CAD build for the part. Positions are in the model's coordinates, mm. A direction names the side the tool comes from. Round coordinates to 2 decimals unless told otherwise and drop trailing zeros. Write each loop counter-clockwise with the first axis right and the second up, starting at its lowest first coordinate (ties: lowest second). Pieces come first, ordered by that corner, then holes. Notation, with made-up numbers: (12.25, 60) -> (33.25, 60) arc R10 ccw to (33.25, 74) -> close; hole circle Ø10 at (56, 49.25). An arc over 180 degrees is marked (long way). Put each result on its own line as item: value. Start each with the question number.
1. Drill centre lines: line 1 (X direction, y = 12.5, z = 46.25); line 2 (X direction, y = -6.5, z = 46.25); line 3 (Y direction, x = 8, z = 40.25). Where is each one in solid material? Low to high. Write a range as from..to.
2. Saw through at C-C on z = 35. List the corners of the cut face in (x, y).
3. Saw through at B-B on x = 0. List the corners of the cut face in (y, z), and give its area (3 significant figures).
4. 3-axis set-ups, long thin cutter, end or side, ignore diameter. For faces 4 (the flat face through (13, 7, 47)), 5 (the flat face through (-9, 0, 41.5)), 6 (the flat face through (-13, 7, 47)), 7 (the flat face through (-11, -7, 39)), 8 (the cylindrical face through (6.384, 7.721, 46.43)): which of +Z, -Z, +X, -X, +Y, -Y reach the whole face in a straight line?
5. Flat gauge pins, fed straight in: P1, Ø15, axis at x = 0, y = -6.5, coming from the -Z side; P2, Ø3, axis at y = 2.5, z = 45, coming from the +X side; P3, Ø1.5, axis at x = -4.5, y = -5, coming from the -Z side; P4, Ø1, axis at x = -5.5, z = 37.5, coming from the +Y side. Where does each tip first touch, or does it go through?
6. Pull direction Z, two halves, no side cores. Call faces 1 (the flat face through (-10, 0, 51.5)), 2 (the flat face through (0, -14, 33)), 3 (the flat face through (12, 0, 46)): pulls with the +Z half, pulls with the -Z half, needs draft (parallel to the pull), parting line crosses it, or undercut.
7. Saw through at D-D on y = -23. List the corners of the cut face in (x, z), and give its area (3 significant figures).
8. Saw through at A-A on y = 0. List the corners of the cut face in (x, z).
from build123d import *

# Parameters (mm, degrees)
BOX005_W                  = 12
BOX005_H                  = 60
BOX005_DEPTH              = 30
BOX006_W                  = 12
BOX006_H                  = 60
BOX006_DEPTH              = 30
BOX004_W                  = 50
BOX004_H                  = 30
BOX004_DEPTH              = 19
BOX004_PLACEMENT_ANGLE    = 15
CYLINDER012_R             = 5.1
CYLINDER012_DEPTH         = 50
CYLINDER007_R             = 7.5
CYLINDER007_DEPTH         = 70
CYLINDER009_R             = 6.5
CYLINDER009_DEPTH         = 70
CYLINDER010_R             = 7.5
CYLINDER010_DEPTH         = 70
CYLINDER011_R             = 6.5
CYLINDER011_DEPTH         = 70
FUSION007_PLACEMENT_ANGLE = 180
CYLINDER008_R             = 5.1
CYLINDER008_DEPTH         = 70
BOX003_W                  = 57
BOX003_H                  = 59
BOX003_DEPTH              = 20
CYLINDER004_R             = 6.35
CYLINDER004_DEPTH         = 50
BOX_W                     = 40
BOX_H                     = 20
BOX_DEPTH                 = 30
BOX_PLACEMENT_ANGLE       = 15
CYLINDER001_R             = 5
CYLINDER001_DEPTH         = 50
CYLINDER006_R             = 6.35
CYLINDER006_DEPTH         = 50
BOX001_W                  = 40
BOX001_H                  = 20
BOX001_DEPTH              = 30
BOX001_PLACEMENT_ANGLE    = 15
CYLINDER005_R             = 5
CYLINDER005_DEPTH         = 50
FUSION003_PLACEMENT_ANGLE = 180
BOX002_W                  = 24
BOX002_H                  = 39
BOX002_DEPTH              = 10


with BuildPart() as cube005:
    # Box005 → Box005 (new body)
    with BuildSketch(Plane(origin=(14, -29, 23), x_dir=(1, 0, 0), z_dir=(0, 0, 1))):
        with Locations((6, 30)):
            Rectangle(BOX005_W, BOX005_H)
    extrude(amount=BOX005_DEPTH)


with BuildPart() as fusion009:
    # Box006 → Box006 (new body)
    with BuildSketch(Plane(origin=(-26, -29, 23), x_dir=(1, 0, 0), z_dir=(0, 0, 1))):
        with Locations((6, 30)):
            Rectangle(BOX006_W, BOX006_H)
    extrude(amount=BOX006_DEPTH)

    # Fusion009: union Cube005
    add(cube005.part)


with BuildPart() as cube004:
    # Box004 → Box004 (new body)
    with BuildSketch(Plane.XY):
        with Locations((25, 15)):
            Rectangle(BOX004_W, BOX004_H)
    extrude(amount=BOX004_DEPTH)


with BuildPart() as cube004_1:
    # Box004 placement: moved
    add(cube004.part.moved(Location((-24, 7.965926, 22.258819))).rotate(Axis((-24, 7.965926, 22.258819), (1, 0, 0)), BOX004_PLACEMENT_ANGLE))


with BuildPart() as obj1:
    # Cylinder012 → Cylinder012 (new body)
    with BuildSketch(Plane(origin=(0, -12.5, -17), x_dir=(1, 0, 0), z_dir=(0, 0, 1))):
        Circle(CYLINDER012_R)
    extrude(amount=CYLINDER012_DEPTH)


with BuildPart() as obj2:
    # Cylinder007 → Cylinder007 (new body)
    with BuildSketch(Plane.XY):
        Circle(CYLINDER007_R)
    extrude(amount=CYLINDER007_DEPTH)


with BuildPart() as fusion006:
    # Cylinder009 → Cylinder009 (new body)
    with BuildSketch(Plane(origin=(0, 6.5, 0), x_dir=(1, 0, 0), z_dir=(0, 0, 1))):
        Circle(CYLINDER009_R)
    extrude(amount=CYLINDER009_DEPTH)

    # Fusion006: union obj2
    add(obj2.part)


with BuildPart() as obj3:
    # Cylinder010 → Cylinder010 (new body)
    with BuildSketch(Plane.XY):
        Circle(CYLINDER010_R)
    extrude(amount=CYLINDER010_DEPTH)


with BuildPart() as fusion008:
    # Cylinder011 → Cylinder011 (new body)
    with BuildSketch(Plane(origin=(0, 6.5, 0), x_dir=(1, 0, 0), z_dir=(0, 0, 1))):
        Circle(CYLINDER011_R)
    extrude(amount=CYLINDER011_DEPTH)

    # Fusion007: union obj3
    add(obj3.part)


with BuildPart() as fusion008_1:
    # Fusion007 placement: moved
    add(fusion008.part.rotate(Axis((0, 0, 0), (0, 0, 1)), FUSION007_PLACEMENT_ANGLE))

    # Fusion008: union Fusion006
    add(fusion006.part)


with BuildPart() as cylinder008:
    # Cylinder008 → Cylinder008 (new body)
    with BuildSketch(Plane(origin=(0, 12.5, 0), x_dir=(1, 0, 0), z_dir=(0, 0, 1))):
        Circle(CYLINDER008_R)
    extrude(amount=CYLINDER008_DEPTH)


with BuildPart() as cube003:
    # Box003 → Box003 (new body)
    with BuildSketch(Plane(origin=(-29.5, -29, 51.5), x_dir=(1, 0, 0), z_dir=(0, 0, 1))):
        with Locations((28.5, 29.5)):
            Rectangle(BOX003_W, BOX003_H)
    extrude(amount=BOX003_DEPTH)


with BuildPart() as obj4:
    # Cylinder004 → Cylinder004 (new body)
    with BuildSketch(Plane.XY):
        Circle(CYLINDER004_R)
    extrude(amount=CYLINDER004_DEPTH)


with BuildPart() as cube:
    # Box → Box (new body)
    with BuildSketch(Plane.XY):
        with Locations((20, 10)):
            Rectangle(BOX_W, BOX_H)
    extrude(amount=BOX_DEPTH)


with BuildPart() as cube_1:
    # Box placement: moved
    add(cube.part.moved(Location((-19.558238, 7, 39.759763))).rotate(Axis((-19.558238, 7, 39.759763), (0, 1, 0)), BOX_PLACEMENT_ANGLE))


with BuildPart() as fusion001:
    # Cylinder001 → Cylinder001 (new body)
    with BuildSketch(Plane(origin=(0, 12.5, 0), x_dir=(1, 0, 0), z_dir=(0, 0, 1))):
        Circle(CYLINDER001_R)
    extrude(amount=CYLINDER001_DEPTH)

    # Fusion: union Cube
    add(cube_1.part)

    # Fusion001: union obj4
    add(obj4.part)


with BuildPart() as obj5:
    # Cylinder006 → Cylinder006 (new body)
    with BuildSketch(Plane.XY):
        Circle(CYLINDER006_R)
    extrude(amount=CYLINDER006_DEPTH)


with BuildPart() as cube001:
    # Box001 → Box001 (new body)
    with BuildSketch(Plane.XY):
        with Locations((20, 10)):
            Rectangle(BOX001_W, BOX001_H)
    extrude(amount=BOX001_DEPTH)


with BuildPart() as cube001_1:
    # Box001 placement: moved
    add(cube001.part.moved(Location((-19.558238, 7, 39.759763))).rotate(Axis((-19.558238, 7, 39.759763), (0, 1, 0)), BOX001_PLACEMENT_ANGLE))


with BuildPart() as fusion004:
    # Cylinder005 → Cylinder005 (new body)
    with BuildSketch(Plane(origin=(0, 12.5, 0), x_dir=(1, 0, 0), z_dir=(0, 0, 1))):
        Circle(CYLINDER005_R)
    extrude(amount=CYLINDER005_DEPTH)

    # Fusion002: union Cube001
    add(cube001_1.part)

    # Fusion003: union obj5
    add(obj5.part)


with BuildPart() as fusion004_1:
    # Fusion003 placement: moved
    add(fusion004.part.rotate(Axis((0, 0, 0), (0, 0, 1)), FUSION003_PLACEMENT_ANGLE))

    # Fusion004: union Fusion001
    add(fusion001.part)


with BuildPart() as cut005:
    # Box002 → Box002 (new body)
    with BuildSketch(Plane(origin=(-12, -13, 41.5), x_dir=(1, 0, 0), z_dir=(0, 0, 1))):
        with Locations((12, 19.5)):
            Rectangle(BOX002_W, BOX002_H)
    extrude(amount=BOX002_DEPTH)

    # Fusion005: union Fusion004
    add(fusion004_1.part)

    # Cut: cut Cube003
    add(cube003.part, mode=Mode.SUBTRACT)

    # Cut001: cut Cylinder008
    add(cylinder008.part, mode=Mode.SUBTRACT)

    # Cut002: cut Fusion008
    add(fusion008_1.part, mode=Mode.SUBTRACT)

    # Cut003: cut obj1
    add(obj1.part, mode=Mode.SUBTRACT)

    # Cut004: cut Cube004
    add(cube004_1.part, mode=Mode.SUBTRACT)

    # Cut005: cut Fusion009
    add(fusion009.part, mode=Mode.SUBTRACT)


solid = cut005.part
Return value:
1. line 1: x = -14..-5.1, 5.1..14
1. line 2: x = -12..-6.5, 6.5..12
1. line 3: y = -27..-7
2. outline: (-14, -27) -> (1.79, -27) -> (1.79, -17.17) arc R5 ccw to (4.75, -10.94) arc R6.5 cw to (-6.48, -7) -> (-14, -7) -> close
3. outline: (-27, 34.52) -> (-17.5, 34.52) -> (-17.5, 33) -> (-13, 33) -> (-13, 51.5) -> (-27, 51.5) -> close; (17.6, 44.51) -> (27, 47.03) -> (27, 51.5) -> (17.6, 51.5) -> close
3. area: 298 mm^2
4. face 4: +Z, -Z, +X
4. face 5: -Z, +X, -X, +Y
4. face 6: +Z, -Z, -X
4. face 7: -Z, -X
4. face 8: +Z, -Z
5. P1: stops at z = 32.51
5. P2: stops at x = 12
5. P3: passes through
5. P4: stops at y = -9
6. face 1: pulls with the +Z half
6. face 2: pulls with the -Z half
6. face 3: needs draft
7. outline: (-14, 30.77) -> (14, 38.27) -> (14, 51.5) -> (-14, 51.5) -> close
7. area: 475 mm^2
8. outline: (-12, 41.5) -> (-7.5, 41.5) -> (-7.5, 51.5) -> (-12, 51.5) -> close; (7.5, 41.5) -> (12, 41.5) -> (12, 51.5) -> (7.5, 51.5) -> close
